Geometry: final body of the model. Coordinates: model frame, mm. A direction names the side the tool comes from. Give positions to 0.01 mm unless a question says otherwise; leave off trailing zeros. Loops run counter-clockwise (first coordinate to the right, second up) from the corner with the lowest first, then second, coordinate; pieces in that order, holes last. Notation, with made-up numbers: (84.5, 6) - (103.5, 6) arc R18 ccw to (103.5, 21) - close; hole circle Ø2 at (75, 0). An arc over 180 degrees is marked (long way). Answer in a Markdown table with one row per item.
Autodesk Inventor part; units mm, degrees
ref_plane "YZ Plane" through (0, 0, 0) normal (1, 0, 0) x (0, 1, 0)
ref_plane "XZ Plane" through (0, 0, 0) normal (0, 1, 0) x (-1, 0, 0)
ref_plane "XY Plane" through (0, 0, 0) normal (0, 0, 1) x (1, 0, 0)
sketch "Эскиз1" plane through (0, 0, 0) normal (1, 0, 0) x (0, 1, 0)
  line L0 (-8, 55) -> (8, 55) construction
  line L1 (8, 55) -> (8, 0)
  line L2 (8, 0) -> (-8, 0) construction
  line L3 (-8, 0) -> (-8, 55)
  line L4 (8, 0) -> (5, 0)
  line L5 (5, 0) -> (5, -27)
  line L6 (5, -27) -> (-5, -27)
  line L7 (-5, -27) -> (-5, 0)
  line L8 (-8, 0) -> (-5, 0)
  line L9 (0, 59) -> (0, -27) construction
  line L10 (8, 55) -> (5, 55)
  line L11 (5, 55) -> (5, 59)
  line L12 (5, 59) -> (0, 59)
  line L13 (-8, 55) -> (-5, 55)
  line L14 (-5, 55) -> (-5, 59)
  line L15 (-5, 59) -> (0, 59)
  line L16 (-2, 37.5) -> (2, 37.5)
  line L17 (2, 37.5) -> (2, 17.5)
  line L18 (2, 17.5) -> (-2, 17.5)
  line L19 (-2, 17.5) -> (-2, 37.5)
  point P0 (0, 0)
  point P1 (2, 27.5)
  point P2 (8, 27.5)
  point P3 (0, 37.5)
  dimension "d0" = 10
  dimension "d1" = 16
  dimension "d2" = 27
  dimension "d3" = 55
  dimension "d4" = 4
  dimension "d7" = 20
  dimension "d8" = 4
extrude "Выдавливание2" add sketch "Эскиз1" along normal blind 4
properties part number "PistonPart4" material "Дерево (вишня)"
Q1. Cut plane D-D (z = -4.5). Output: boundary loops of the cut face in (x, y), and give its area (3 significant figures).
Check values:
| item | result |
|---|---|
| outline | (0, -5) - (4, -5) - (4, 5) - (0, 5) - close |
| area | 40.0 mm² |
Q2. Draft query along Y for faces 1 (the flat face through (2, -7, 0)), 2 (the flat face through (2, -2, 27)), 3 (the flat face through (2, -5, 57)), 4 (the flat face through (2, 0, 17.5)). Return one class per face: pulls with the +Y half, pulls with the -Y half, needs draft (parallel to the pull), parting line crosses it, or undercut.
Check values:
| item | result |
|---|---|
| face 1 | needs draft |
| face 2 | undercut |
| face 3 | pulls with the -Y half |
| face 4 | undercut |
Q3. First-contact query: pin 1 (2 mm diameter, centred on x = 3, y = -6.5, fed in from -Z); pin 2 (2 mm diameter, centred on x = 1.5, z = -11, fed in from +Y). Flat tips, straight axial feed; report the tip coordinate or a pass-through.
Check values:
| item | result |
|---|---|
| pin 1 | z = 0 |
| pin 2 | y = 5 |
Q4. Cut plane C-C (x = 1.75). Output: boundary loops of the cut face in (y, z), and give its area (3 significant figures).
Check values:
| item | result |
|---|---|
| outline | (-8, 0) - (-5, 0) - (-5, -27) - (5, -27) - (5, 0) - (8, 0) - (8, 55) - (5, 55) - (5, 59) - (-5, 59) - (-5, 55) - (-8, 55) - close; hole (-2, 17.5) - (2, 17.5) - (2, 37.5) - (-2, 37.5) - close |
| area | 1,110 mm² |
Q5. Cut plane A-A (y = 1.25). Output: boundary loops of the cut face in (x, z).
Check values:
| item | result |
|---|---|
| outline | (0, -27) - (4, -27) - (4, 17.5) - (0, 17.5) - close; (0, 37.5) - (4, 37.5) - (4, 59) - (0, 59) - close |
Q6. Cut plane B-B (z = 25.5). Output: boundary loops of the cut face in (x, y).
Check values:
| item | result |
|---|---|
| outline | (0, -8) - (4, -8) - (4, -2) - (0, -2) - close; (0, 2) - (4, 2) - (4, 8) - (0, 8) - close |
Q7. Material intervals for line 1 along Y through (x, z) = (3.3, 32); line 2 along Z through (x, y) = (2.35, -1.5); line 3 along Y through (x, z) = (1.4, -3.5), sorted ascending.
Check values:
| item | result |
|---|---|
| line 1 | -8 to -2, 2 to 8 |
| line 2 | -27 to 17.5, 37.5 to 59 |
| line 3 | -5 to 5 |
Q8. Reachability of faces 5 (the flat face through (2, -5, -14)), 6 (the flat face through (2, 7, 55)), 7 (the flat face through (2, -7, 55)), 8 (the flat face through (2, 2, 28)) from +Z, -Z, +X, -X, +Y, -Y: full face, straight path, thin tool, end or side. Return the list, or none.
Check values:
| item | result |
|---|---|
| face 5 | -Z, +X, -X, -Y |
| face 6 | +Z, +X, -X, +Y |
| face 7 | +Z, +X, -X, -Y |
| face 8 | +X, -X |
